```python
from build123d import *

# Parameters (mm, degrees)
MAIN_EXTRUSION_DEPTH    = 4
CONG_1_R                = 5
ESQUISSE1_R             = 1
ENL_V_MAT_EXTRU_1_DEPTH = 257.850637531
D_GAGEMENT_M31_D        = 3.4
ESQUISSE4_R             = 1
ESQUISSE4_R_2           = 1.5
ESQUISSE4_W             = 53
ESQUISSE4_H             = 15
ENL_V_MAT_EXTRU_2_DEPTH = 257.850637531
D_GAGEMENT_M32_D        = 3.4
ESQUISSE7_W             = 90
ESQUISSE7_H             = 16
ESQUISSE7_W_2           = 38
ESQUISSE7_H_2           = 22
ESQUISSE7_W_3           = 16
ESQUISSE7_H_3           = 25
ESQUISSE7_W_4           = 15
ESQUISSE7_H_4           = 45
ENL_V_MAT_EXTRU_3_DEPTH = 4
CONG_2_R                = 3


with BuildPart() as part:
    # Main scetch → Main extrusion (new body)
    with BuildSketch(Plane(origin=(0, 0, 0), x_dir=(1, 0, 0), z_dir=(0, 1, 0))):
        Polygon((-92.5, 0), (92.5, 0), (132.5, 40), (132.5, 220), (102.5, 220), (85.179491924, 190), (-85.179491924, 190), (-102.5, 220), (-132.5, 220), (-132.5, 40), align=None)
    extrude(amount=MAIN_EXTRUSION_DEPTH)

    # Congé1
    cong_1_edges = [part.edges().sort_by_distance(p)[0] for p in [
        (132.5, 2, -220),
        (132.5, 2, -40),
        (92.5, 2, 0),
        (-92.5, 2, 0),
        (-132.5, 2, -40),
        (-132.5, 2, -220),
        (-102.5, 2, -220),
        (-85.179491924, 2, -190),
        (85.179491924, 2, -190),
        (102.5, 2, -220),
    ]]
    fillet(cong_1_edges, radius=CONG_1_R)

    # Esquisse1 → Enlèv. mat.-Extru.1 (cut, through all)
    with BuildSketch(Plane(origin=(0, 4, 0), x_dir=(1, 0, 0), z_dir=(0, 1, 0))):
        with Locations(Location((70, 8, 0), (0, 0, 270))):
            Circle(ESQUISSE1_R)
        with Locations(Location((124.5, 70, 0), (0, 0, 270))):
            Circle(ESQUISSE1_R)
        with Locations(Location((124.5, 212, 0), (0, 0, 270))):
            Circle(ESQUISSE1_R)
        with Locations(Location((-124.5, 212, 0), (0, 0, 90))):
            Circle(ESQUISSE1_R)
        with Locations(Location((-124.5, 70, 0), (0, 0, 90))):
            Circle(ESQUISSE1_R)
        with Locations(Location((-70, 8, 0), (0, 0, 90))):
            Circle(ESQUISSE1_R)
    extrude(amount=-ENL_V_MAT_EXTRU_1_DEPTH, mode=Mode.SUBTRACT)

    # Dégagement M31 (through all)
    with Locations(Plane(origin=(0, 4, 0), x_dir=(1, 0, 0), z_dir=(0, 1, 0))):
        with Locations((-124.5, 212), (-124.5, 70), (-70, 8), (70, 8), (124.5, 70), (124.5, 212)):
            Hole(D_GAGEMENT_M31_D / 2)

    # Esquisse4 → Enlèv. mat.-Extru.2 (cut, through all)
    with BuildSketch(Plane(origin=(0, 4, 0), x_dir=(1, 0, 0), z_dir=(0, 1, 0))):
        with Locations(Location((72.5, 167, 0), (0, 0, 270))):
            Circle(ESQUISSE4_R)
        with Locations(Location((41.5, 142, 0), (0, 0, 270))):
            Circle(ESQUISSE4_R)
        with Locations(Location((107.5, 155, 0), (0, 0, 270))):
            Circle(ESQUISSE4_R)
        with Locations(Location((127.5, 195, 0), (0, 0, 270))):
            Circle(ESQUISSE4_R)
        with Locations(Location((112, 120, 0), (0, 0, 270))):
            Circle(ESQUISSE4_R)
        with Locations(Location((112.5, 90, 0), (0, 0, 270))):
            Circle(ESQUISSE4_R)
        with Locations(Location((17.2, 120, 0), (0, 0, 270))):
            Circle(ESQUISSE4_R)
        with Locations(Location((17.2, 90, 0), (0, 0, 270))):
            Circle(ESQUISSE4_R)
        with Locations(Location((47.5, 88, 0), (0, 0, 270))):
            Circle(ESQUISSE4_R)
        with Locations(Location((57.5, 50, 0), (0, 0, 270))):
            Circle(ESQUISSE4_R)
        with Locations(Location((97.5, 50, 0), (0, 0, 270))):
            Circle(ESQUISSE4_R)
        with Locations(Location((52.5, 20, 0), (0, 0, 270))):
            Circle(ESQUISSE4_R)
        with Locations(Location((-10, 85, 0), (0, 0, 270))):
            Circle(ESQUISSE4_R)
        with Locations(Location((-72.5, 20, 0), (0, 0, 270))):
            Circle(ESQUISSE4_R)
        with Locations(Location((107.5, 195, 0), (0, 0, 270))):
            Circle(ESQUISSE4_R)
        with Locations(Location((-47.5, 78, 0), (0, 0, 270))):
            Circle(ESQUISSE4_R)
        with Locations(Location((25.14, 78, 0), (0, 0, 270))):
            Circle(ESQUISSE4_R)
        with Locations(Location((-47.5, 19.07, 0), (0, 0, 270))):
            Circle(ESQUISSE4_R)
        with Locations(Location((25.109569617, 18.82, 0), (0, 0, 270))):
            Circle(ESQUISSE4_R)
        with Locations(Location((-125, 146, 0), (0, 0, 270))):
            Circle(ESQUISSE4_R)
        with Locations(Location((-125, 84, 0), (0, 0, 270))):
            Circle(ESQUISSE4_R)
        with Locations(Location((-31, 7.5, 0), (0, 0, 270))):
            Circle(ESQUISSE4_R)
        with Locations(Location((31, 7.5, 0), (0, 0, 270))):
            Circle(ESQUISSE4_R)
        with Locations(Location((125, 146, 0), (0, 0, 270))):
            Circle(ESQUISSE4_R)
        with Locations(Location((125, 84, 0), (0, 0, 270))):
            Circle(ESQUISSE4_R)
        with Locations(Location((50.5, 182.5, 0), (0, 0, 270))):
            Circle(ESQUISSE4_R)
        with Locations(Location((112.5, 182.5, 0), (0, 0, 270))):
            Circle(ESQUISSE4_R)
        with Locations(Location((-112.5, 182.5, 0), (0, 0, 270))):
            Circle(ESQUISSE4_R)
        with Locations(Location((-50.5, 182.5, 0), (0, 0, 270))):
            Circle(ESQUISSE4_R)
        with Locations(Location((-45, 185, 0), (0, 0, 270))):
            Circle(ESQUISSE4_R)
        with Locations(Location((-45, 157.5, 0), (0, 0, 270))):
            Circle(ESQUISSE4_R)
        with Locations(Location((-68.5, 157.5, 0), (0, 0, 270))):
            Circle(ESQUISSE4_R)
        with Locations(Location((-92, 157.5, 0), (0, 0, 270))):
            Circle(ESQUISSE4_R)
        with Locations(Location((-92, 185, 0), (0, 0, 270))):
            Circle(ESQUISSE4_R)
        with Locations(Location((126, 50, 0), (0, 0, 270))):
            Circle(ESQUISSE4_R_2)
        with Locations(Location((-60, 6.5, 0), (0, 0, 270))):
            Circle(ESQUISSE4_R_2)
        with Locations(Location((60, 6.5, 0), (0, 0, 270))):
            Circle(ESQUISSE4_R_2)
        with Locations(Location((-126, 50, 0), (0, 0, 270))):
            Circle(ESQUISSE4_R_2)
        with Locations(Location((-126, 200, 0), (0, 0, 270))):
            Circle(ESQUISSE4_R_2)
        with Locations(Location((-81.5, 65, 0), (0, 0, 270))):
            Circle(ESQUISSE4_R_2)
        with Locations(Location((-81.5, 15, 0), (0, 0, 270))):
            Circle(ESQUISSE4_R_2)
        with Locations(Location((-101.5, 40, 0), (0, 0, 270))):
            Circle(ESQUISSE4_R_2)
        with Locations((0, 7.5)):
            Rectangle(ESQUISSE4_W, ESQUISSE4_H)
    extrude(amount=-ENL_V_MAT_EXTRU_2_DEPTH, mode=Mode.SUBTRACT)

    # Dégagement M32 (through all)
    with Locations(Plane(origin=(0, 4, 0), x_dir=(1, 0, 0), z_dir=(0, 1, 0))):
        with Locations((17.2, 120), (41.5, 142), (72.5, 167), (107.5, 155), (127.5, 195), (112, 120), (112.5, 90), (47.5, 88), (17.2, 90), (57.5, 50), (97.5, 50), (-10, 85), (-72.5, 20), (52.5, 20), (107.5, 195), (-47.5, 78), (25.14, 78), (-47.5, 19.07), (25.109569617, 18.82), (-125, 146), (-125, 84), (-31, 7.5), (31, 7.5), (125, 146), (125, 84), (-112.5, 182.5), (-50.5, 182.5), (50.5, 182.5), (112.5, 182.5), (-92, 185), (-92, 157.5), (-68.5, 157.5), (-45, 157.5), (-45, 185), (126, 50), (-60, 6.5), (60, 6.5), (-126, 200), (-126, 50), (-81.5, 65), (-81.5, 15), (-101.5, 40)):
            Hole(D_GAGEMENT_M32_D / 2)

    # Esquisse7 → Enlèv. mat.-Extru.3 (cut)
    with BuildSketch(Plane(origin=(0, 4, 0), x_dir=(1, 0, 0), z_dir=(0, 1, 0))):
        with Locations((-32.5, 123)):
            Rectangle(ESQUISSE7_W, ESQUISSE7_H)
        Polygon((40.5, 115), (98.5, 115), (98.5, 168), (83.5, 168), (83.5, 131), (40.5, 131), align=None)
        with Locations((79.5, 31)):
            Rectangle(ESQUISSE7_W_2, ESQUISSE7_H_2)
        with Locations((-110.5, 162.5)):
            Rectangle(ESQUISSE7_W_3, ESQUISSE7_H_3)
        Polygon((-71.5, 28), (-55.5, 28), (-55.5, 82), (-21.5, 82), (-21.5, 97), (-71.5, 97), (-71.5, 83), align=None)
        with Locations((39, 49.32)):
            Rectangle(ESQUISSE7_W_4, ESQUISSE7_H_4)
    extrude(amount=-ENL_V_MAT_EXTRU_3_DEPTH, mode=Mode.SUBTRACT)

    # Congé2
    cong_2_edges = [part.edges().sort_by_distance(p)[0] for p in [
        (-102.5, 2, -150),
        (-102.5, 2, -175),
        (-118.5, 2, -175),
        (-118.5, 2, -150),
        (83.5, 2, -168),
        (83.5, 2, -131),
        (40.5, 2, -131),
        (40.5, 2, -115),
        (98.5, 2, -115),
        (98.5, 2, -168),
        (98.5, 2, -20),
        (98.5, 2, -42),
        (60.5, 2, -42),
        (60.5, 2, -20),
        (-55.5, 2, -28),
        (-55.5, 2, -82),
        (-21.5, 2, -82),
        (-21.5, 2, -97),
        (-71.5, 2, -97),
        (-71.5, 2, -28),
        (46.5, 2, -26.82),
        (46.5, 2, -71.82),
        (31.5, 2, -71.82),
        (31.5, 2, -26.82),
        (12.5, 2, -115),
        (12.5, 2, -131),
        (-77.5, 2, -131),
        (-77.5, 2, -115),
    ]]
    fillet(cong_2_edges, radius=CONG_2_R)


solid = part.part
```
Here's how the part is built. I have some questions about the finished solid (model axes, mm). A direction names the side the tool comes from. Give positions to 0.01 mm unless a question says otherwise; leave off trailing zeros. Put each result on its own line as item: value. Start each with the question number.
Item 1: Will this pin go through, and if not, where does the flat tip stop? pin 1 (1.5 mm diameter, centred on x = 103.5, y = 2, fed in from +Z).
Item 2: On a 3-axis mill with a long thin cutter (end or side, diameter ignored), from which of +Z, -Z, +X, -X, +Y, -Y can I reach the whole of each face in a straight line? I mean faces 1 (the flat face through (-2, 0, -112)), 2 (the flat face through (-93.739, 1.972, -204.825)). Say none if no direction works.
Item 3: I need wall thicknesses on L1, parallel to X at y = 2.1, z = -120; L2, parallel to X at y = 2.2, z = -88; L3, parallel to Z at x = -27, y = 0.4. Which ranges of each line are inside material? Lowest first, please. Write a range as from..to.
Item 4: If we section it at A-A, the plane y = 1.6: Count the separate pieces of the cut face and the enclosed holes in it, then the cut area to 3 significant figures.
Item 5: Thinking about a two-plate mould opening in X: for faces 3 (the flat face through (-112.8, 2, -20.3)), 4 (the flat face through (-2, 4, -112)), 5 (the flat face through (93.941, 1.972, -205.175)), 6 (the flat face through (112.2, 2, -19.7)), which applies, +X half, -X half, draft (parallel to the pull), parting line (faces both ways), or undercut?
Values:
1. pin 1: z = -10.25
2. face 1: +Z, -Z, +X, -X, -Y
2. face 2: -Z, +Y, -Y
3. L1: -132.5..-77.5, 12.5..15.5, 18.9..40.5, 98.5..110.3, 113.7..132.5
3. L2: -132.5..-71.5, -21.5..45.8, 49.2..132.5
3. L3: -190..-131, -115..-97, -82..0
4. separate pieces: 1
4. enclosed holes: 54
4. area: 43,400 mm²
5. face 3: -X half
5. face 4: draft
5. face 5: undercut
5. face 6: +X half
